Autodesk Inventor part; units mm, degrees
ref_plane "YZ Plane" through (0, 0, 0) normal (1, 0, 0) x (0, 1, 0)
ref_plane "XZ Plane" through (0, 0, 0) normal (0, 1, 0) x (-1, 0, 0)
ref_plane "XY Plane" through (0, 0, 0) normal (0, 0, 1) x (1, 0, 0)
sketch "Sketch1" plane through (0, 0, 0) normal (0, 1, 0) x (-1, 0, 0)
  line L0 (0, 0) -> (-60, 0)
  line L1 (-60, 0) -> (-60, -200)
  line L2 (-60, -200) -> (0, -200)
  line L3 (0, -200) -> (0, 0)
  dimension "d0" = 60
  dimension "d1" = 200
extrude "Base" add sketch "Sketch1" along normal blind 3
sketch "Sketch4" plane through (0, 3, 0) normal (0, 1, 0) x (1, 0, 0)
  line L0 (0, 0) -> (60, 0)
  line L1 (60, 0) -> (60, 200)
  line L2 (60, 200) -> (0, 200)
  line L3 (0, 200) -> (0, 0)
  line L4 (3, 3) -> (57, 3)
  line L5 (57, 3) -> (57, 197)
  line L6 (57, 197) -> (3, 197)
  line L7 (3, 197) -> (3, 3)
  line L8 (19.7, 0) -> (40.3, 0)
  line L9 (40.3, 0) -> (40.3, 3)
  line L10 (40.3, 3) -> (19.7, 3)
  line L11 (19.7, 3) -> (19.7, 0)
  point P0 (30, 0)
  point P1 (30, 3)
  dimension "d6" = 3
  dimension "d7" = 20.6
extrude "Paredes" add sketch "Sketch4" along normal blind 10 contours L3 L2 L1 L0 L9 L4 L5 L6 L7 L11
sketch "Sketch5" plane through (0, 3, 0) normal (0, 1, 0) x (1, 0, 0)
  line L0 (27.5, 0) -> (32.5, 0)
  line L1 (32.5, 0) -> (32.5, 197)
  line L2 (32.5, 197) -> (27.5, 197)
  line L3 (27.5, 197) -> (27.5, 0)
  line L4 (19.7, 0) -> (40.3, 0)
  line L5 (57, 197) -> (3, 197)
  point P0 (0, 0)
  point P1 (30, 0)
  point P2 (30, 197)
  dimension "d10" = 5
extrude "Canal" cut sketch "Sketch5" against normal blind 1.5
sketch "Sketch6" plane through (0, 3, 0) normal (0, 1, 0) x (1, 0, 0)
  line L0 (6.5, 3.0083) -> (6.5, 197)
  line L1 (27.5, 197) -> (3, 197)
  line L2 (3, 197) -> (3, 3)
  line L3 (3, 3) -> (19.7, 3)
  point P0 (0, 0)
  point P1 (6.5, 53)
  point P2 (6.5, 147)
  dimension "d13" = 3.5
  dimension "d14" = 50
  dimension "d15" = 50
hole "Agujeros" at (6.5, 3, -53) at (6.5, 3, -147) direction (0, -1, 0) diameter 2 end through all
ref_plane "Mitad" through (30, 3, -3) normal (1, 0, 0) x (0, 0, -1)
sketch "Sketch9" plane through (0, 3, 0) normal (0, 1, 0) x (1, 0, 0)
  line L0 (9.7, 55) -> (14.7, 55)
  line L1 (14.7, 55) -> (14.7, 145)
  line L2 (14.7, 145) -> (9.7, 145)
  line L3 (9.7, 145) -> (9.7, 55)
  line L4 (30, 240) -> (30, -40)
  line L5 (3, 197) -> (3, 3)
  line L6 (3, 100) -> (57, 100)
  line L7 (57, 197) -> (57, 3)
  point P0 (0, 0)
  point P1 (14.7, 100)
  dimension "d23" = 15.3
  dimension "d24" = 90
  dimension "d25" = 5
extrude "Soporte base" add sketch "Sketch9" along normal blind 4
chamfer "Chaflán soporte" distance 2.5 angle 45 2 edges at (14.7, 5, -55) (14.7, 5, -145)
sketch "Sketch10" plane through (0, 7, 0) normal (0, 1, 0) x (1, 0, 0)
  line L0 (9.7, 95) -> (14.7, 95)
  line L1 (14.7, 95) -> (14.7, 105)
  line L2 (14.7, 105) -> (9.7, 105)
  line L3 (9.7, 105) -> (9.7, 95)
  line L4 (9.7, 145) -> (9.7, 55)
  line L5 (14.7, 57.5) -> (14.7, 142.5)
  point P0 (0, 0)
  point P1 (9.7, 100)
  point P2 (14.7, 100)
  dimension "d31" = 10
extrude "Soporte tope" add sketch "Sketch10" along normal blind 5
mirror "Segundo soporte" about plane through (30, 3, -3) normal (1, 0, 0) of "Soporte base", "Chaflán soporte", "Soporte tope"
equation "\"d0\" = base_ancho"
equation "\"d1\" = base_largo"
equation "\"d2\" = base_alto"
equation "\"d6\" = muros_grosor"
equation "\"d7\" = hoja_ancho + 2 * margen"
equation "\"d8\" = muros_alto"
equation "\"d10\" = rail_grosor"
equation "\"d11\" = rail_alto"
equation "\"d13\" = base_agujeros_separacion"
equation "\"d16\" = base_agujeros_diametro"
equation "\"d21\" = d14"
equation "\"d23\" = 0.5 * hoja_ancho_total + margen"
equation "\"d24\" = deslizador_soporte_largo"
equation "\"d25\" = deslizador_soporte_ancho"
equation "\"d26\" = deslizador_soporte_alto"
equation "\"d28\" = 0.5 * deslizador_soporte_ancho"
equation "\"d31\" = deslizador_tope_largo"
equation "\"d32\" = deslizador_tope_alto"
equation "\"margen\" = 0.3"
equation "\"hoja_stop_largo\" = 5"
equation "\"hoja_stop_saliente\" = 5"
equation "\"hoja_stop_posicion\" = 5"
equation "\"hoja_alto\" = 3"
equation "\"rail_grosor\" = 5"
equation "\"base_alto\" = 3"
equation "\"base_ancho\" = 60"
equation "\"base_largo\" = 200"
equation "\"muros_alto\" = 10"
equation "\"muros_grosor\" = 3"
equation "\"rail_alto\" = 1.5"
equation "\"hoja_stop_biselado\" = 2"
equation "\"hoja_cola_biselado\" = 1"
equation "\"hoja_filo_biselado\" = 0.5"
equation "\"deslizador_soporte_alto\" = 4"
equation "\"deslizador_soporte_ancho\" = 5"
equation "\"deslizador_tope_alto\" = 5"
equation "\"deslizador_soporte_largo\" = 90"
equation "\"deslizador_tope_largo\" = 10"
equation "\"deslizador_alto\" = 3"
equation "\"tirador_agarre_largo\" = 3"
equation "\"deslizador_saliente\" = 5"
equation "\"deslizador_largo\" = 144"
equation "\"deslizador_interruptor_largo\" = 5"
equation "\"deslizador_interruptor_ancho\" = 7"
equation "\"traba_largo\" = 39"
equation "\"traba_diametro\" = 5"
equation "\"traba_ancho\" = 3"
equation "\"traba_top_alto\" = 3"
equation "\"traba_alto\" = 4"
equation "\"traba_top_largo\" = 5"
equation "\"traba_diametro_perforacion\" = 2"
equation "\"base_agujeros_distancia\" = 50"
equation "\"base_agujeros_separacion\" = 3.5"
equation "\"base_agujeros_diametro\" = 2"
properties part number "Base"
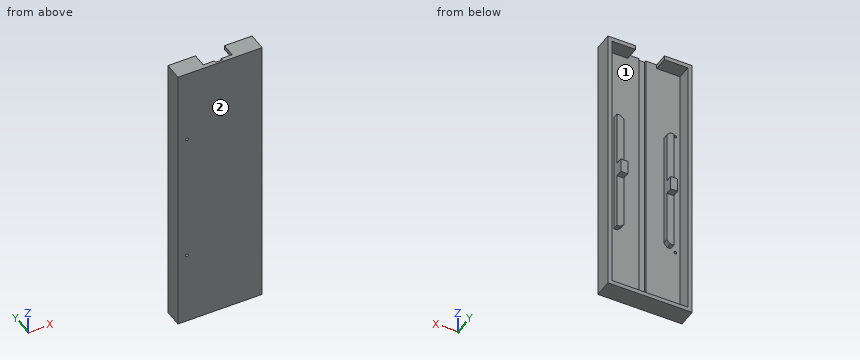
Input: part model. Units: mm. Frame: model coordinates. Face numbers are marked on the shaded views. Coordinates: 2 decimals unless noted, no trailing zeros. Loops run counter-clockwise (first coordinate to the right, second up) from the corner with the lowest first, then second, coordinate; pieces in that order, holes last. Notation, with made-up numbers: M 1.25,38 L 25.25,38 A20 cw 25.25,77 Z; hole C 47,27.25 d5. An arc over 180 degrees is marked long. Use a Markdown table: item, result. Add a question column.
1) Section B-B, the plane x = 52. Return the cut outline in (y, z).
2) Line query: L1, parallel to X at y = 1.6, z = -53; L2, parallel to Z at x = 12, y = 4; L3, parallel to X at y = 6.25, z = -86. Output: solid intervals per line, ascending. Write a range as from..to.
3) Section C-C, the plane z = -178. Return the cut outline in (x, y).
4) Pin query (flat end, axial travel): P1, Ø2, axis at x = 7, z = -75.5, coming from the +Y side; P2, Ø5.5, axis at x = 47, z = -100.5, coming from the +Y side; P3, Ø7.5, axis at x = 11, z = -112.5, coming from the +Y side. Return the tip coordinate at first contact, or that it passes through.
5) Section D-D, the plane x = 37. Return the cut outline in (y, z).
6) Section A-A, the plane z = -73. Return the cut outline in (x, y).
7) Draft query along Z for the marked faces 1 and 2. Return one class per face: +Z half, -Z half, draft (parallel to the pull), parting line (faces both ways), or undercut.
Answer below:
| question | item | result |
|---|---|---|
| 1 | outline | M 0,-200 L 13,-200 L 13,-197 L 3,-197 L 3,-3 L 13,-3 L 13,0 L 0,0 Z |
| 2 | L1 | 0..5.5, 7.5..27.5, 32.5..60 |
| 2 | L2 | -200..-197, -145..-55, -3..0 |
| 2 | L3 | 0..3, 9.7..14.7, 45.3..50.3, 57..60 |
| 3 | outline | M 0,0 L 60,0 L 60,13 L 57,13 L 57,3 L 32.5,3 L 32.5,1.5 L 27.5,1.5 L 27.5,3 L 3,3 L 3,13 L 0,13 Z |
| 4 | P1 | y = 3 |
| 4 | P2 | y = 12 |
| 4 | P3 | y = 7 |
| 5 | outline | M 0,-200 L 13,-200 L 13,-197 L 3,-197 L 3,0 L 0,0 Z |
| 6 | outline | M 0,0 L 60,0 L 60,13 L 57,13 L 57,3 L 50.3,3 L 50.3,7 L 45.3,7 L 45.3,3 L 32.5,3 L 32.5,1.5 L 27.5,1.5 L 27.5,3 L 14.7,3 L 14.7,7 L 9.7,7 L 9.7,3 L 3,3 L 3,13 L 0,13 Z |
| 7 | face 1 | undercut |
| 7 | face 2 | draft |
